Read the model definition and answer for the solid it produces. Units are mm, in the model's axes. Coordinates: 2 decimals unless noted, no trailing zeros. Loops run counter-clockwise (first coordinate to the right, second up) from the corner with the lowest first, then second, coordinate; pieces in that order, holes last. Notation, with made-up numbers: (42, 43) - (73, 43) arc R20 cw to (73, 76) - close; hole circle Ø2 at (-38, 33). An arc over 180 degrees is marked (long way). Use one line per item in the form item = value. Start each with the question number.
1) A cutting plane is placed at D-D (y = -125). Give the vertices of the cut face in (x, z).
2) A cutting plane is placed at B-B (z = 3.8). Give the vertices of the cut face in (x, y), and give its area (3 significant figures).
3) A cutting plane is placed at A-A (y = -29). Give the vertices of the cut face in (x, z).
4) Consider line 1 (Y direction, x = 0, z = 1.2); line 2 (Y direction, x = 13, z = 4.2); line 3 (X direction, y = 37.5, z = 1.1). Determine where each line is inside the solid, lowest interval first.
5) A cutting plane is placed at C-C (x = 15). Give the vertices of the cut face in (y, z), and give its area (3 significant figures).
6) Each of these flat-tipped pins is pushed along its axis until it touches: P1, Ø3, axis at x = -75, y = 0, coming from the -Z side; P2, Ø1, axis at x = 47, z = 1.5, coming from the +Y side; P3, Ø3, axis at x = 122.5, z = 0.5, coming from the -Y side; P4, Ø1.5, axis at y = -38.5, z = 2, coming from the +X side. Where does it stop, or does it pass through?
Autodesk Inventor part; units mm, degrees
ref_plane "YZ Plane" through (0, 0, 0) normal (1, 0, 0) x (0, 1, 0)
ref_plane "XZ Plane" through (0, 0, 0) normal (0, 1, 0) x (-1, 0, 0)
ref_plane "XY Plane" through (0, 0, 0) normal (0, 0, 1) x (1, 0, 0)
sketch "Sketch1" plane through (0, 0, 0) normal (0, 0, 1) x (1, 0, 0)
  circle A0 centre (0, 0) radius 150
  circle A1 centre (0, 0) radius 100
  circle A2 centre (0, 0) radius 155
  circle A3 centre (0, -125) radius 25
  circle A4 centre (0, 0) radius 87.5
  circle A5 centre (0, 0) radius 75
  circle A6 centre (0, 0) radius 50
  circle A7 centre (75, 0) radius 2.5
  circle A8 centre (0, -75) radius 2.5
  circle A9 centre (0, 75) radius 2.5
  circle A10 centre (-75, 0) radius 2.5
  point P0 (0, -150)
  point P1 (0, -100)
  dimension "d0" = 300
  dimension "d1" = 200
  dimension "d2" = 310
  dimension "d3" = 50
  dimension "d8" = 175
  dimension "d9" = 150
  dimension "d10" = 100
  dimension "d11" = 5
  dimension "d12" = 5
  dimension "d13" = 5
  dimension "d14" = 5
extrude "Extrusion1" add sketch "Sketch1" along normal blind 5 contours A1 | A0 | A2 | A4 | A7 A5 A8 A10 A9
equation "\"d0\" = 6 * Product_dia"
equation "\"d1\" = 4 * Product_dia"
equation "\"d3\" = Product_dia"
equation "\"d8\" = 3.5 * Product_dia"
equation "\"d12\" = d11"
equation "\"d13\" = d11"
equation "\"d14\" = d11"
equation "\"Product_dia\" = 50"
equation "\"GridTotalSize\" = 63"
equation "\"GridBorderThickness\" = 5"
equation "\"GridBorderFillets\" = 7"
equation "\"BaseTotalWidth\" = 352"
equation "\"GridProcutClearance\" = 3"
equation "\"ProductBaseHeight\" = 35"
properties material "Steel, Paint Finish, Blue"
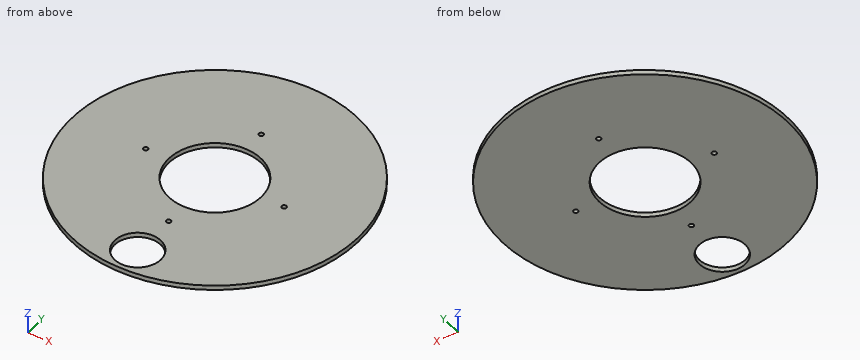
Found:
q1.outline = (-91.65, 0) - (-25, 0) - (-25, 5) - (-91.65, 5) - close; (25, 0) - (91.65, 0) - (91.65, 5) - (25, 5) - close
q2.outline = circle Ø310 at (0, 0); hole circle Ø5 at (-75, 0); hole circle Ø100 at (0, 0); hole circle Ø50 at (0, -125); hole circle Ø5 at (0, -75); hole circle Ø5 at (0, 75); hole circle Ø5 at (75, 0)
q2.area = 65,600 mm^2
q3.outline = (-152.26, 0) - (-40.73, 0) - (-40.73, 5) - (-152.26, 5) - close; (40.73, 0) - (152.26, 0) - (152.26, 5) - (40.73, 5) - close
q4.line_1 = -155 to -150, -100 to -77.5, -72.5 to -50, 50 to 72.5, 77.5 to 155
q4.line_2 = -154.45 to -146.35, -103.65 to -48.28, 48.28 to 154.45
q4.line_3 = -150.4 to -33.07, 33.07 to 150.4
q5.outline = (-154.27, 0) - (-145, 0) - (-145, 5) - (-154.27, 5) - close; (-105, 0) - (-47.7, 0) - (-47.7, 5) - (-105, 5) - close; (47.7, 0) - (154.27, 0) - (154.27, 5) - (47.7, 5) - close
q5.area = 866 mm^2
q6.P1 = through
q6.P2 = 147.86
q6.P3 = -96.87
q6.P4 = 150.33
